Print and shaded views of the part. All mm, measured from the part's lowest x, y and z. Give positions to 0.01 mm unless a question says otherwise; leave off trailing zeros. Loops run counter-clockwise (first coordinate to the right, second up) from the corner with the lowest first, then second, coordinate; pieces in that order, holes last. Notation, with made-up numbers: M -20.5,37.5 L 24.5,37.5 A9 cw 24.5,42.5 Z; hole C -25,32 d11. An arc over 180 degrees is marked long. Answer in a Markdown table with one row per item.
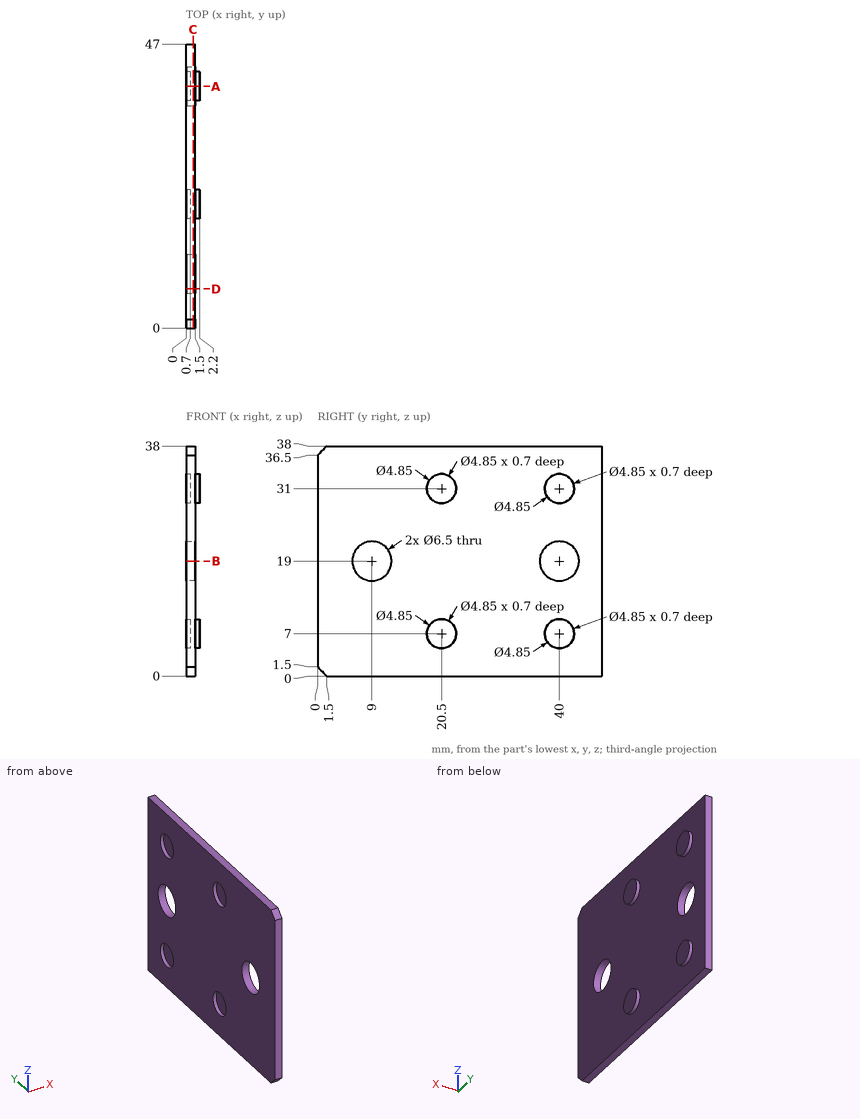
(1) Saw through at A-A, the plane y = 40. Give the cut face in (x, z) (3 decimals), and give its area (4 significant figures).
Established:
| item | result |
|---|---|
| outline | M 0,0 L 1.5,0 L 1.5,4.575 L 2.2,4.575 L 2.2,9.425 L 1.5,9.425 L 1.5,15.75 L 0,15.75 L 0,9.425 L 0.7,9.425 L 0.7,4.575 L 0,4.575 Z; M 0,22.25 L 1.5,22.25 L 1.5,28.575 L 2.2,28.575 L 2.2,33.425 L 1.5,33.425 L 1.5,38 L 0,38 L 0,33.425 L 0.7,33.425 L 0.7,28.575 L 0,28.575 Z |
| area | 47.25 mm2 |
(2) Flat gauge pins, fed straight in: P1, Ø4, axis at y = 40.5, z = 9.5, coming from the +X side; P2, Ø1.5, axis at y = 41, z = 30, coming from the -X side; P3, Ø3, axis at y = 8, z = 13, coming from the +X side. Where does each tip first touch, or does it go through?
Established:
| item | result |
|---|---|
| P1 | stops at x = 2.2 |
| P2 | stops at x = 0.7 |
| P3 | stops at x = 1.5 |
(3) Wall check: L1, parallel to Y at x = 0.45, z = 7 (3 decimals); L2, parallel to Y at x = 2.1, z = 31 (3 decimals); L3, parallel to X at y = 25, z = 30.5. Give the ranges that are in metal, low to high.
Established:
| item | result |
|---|---|
| L1 | y = 0 to 18.075, 22.925 to 37.575, 42.425 to 47 |
| L2 | y = 18.075 to 22.925, 37.575 to 42.425 |
| L3 | x = 0 to 1.5 |
(4) Saw through at D-D, the plane y = 6.5. Give the cut face in (x, z), and give its area (3 significant figures).
Established:
| item | result |
|---|---|
| outline | M 0,0 L 1.5,0 L 1.5,16.92 L 0,16.92 Z; M 0,21.08 L 1.5,21.08 L 1.5,38 L 0,38 Z |
| area | 50.8 mm2 |
(5) Saw through at C-C, the plane x = 1.15. Give the cut face in (y, z), and give its area (3 significant figures).
Established:
| item | result |
|---|---|
| outline | M 0,1.5 L 1.5,0 L 47,0 L 47,38 L 1.5,38 L 0,36.5 Z; hole C 9,19 d6.5; hole C 40,19 d6.5 |
| area | 1,720 mm2 |
(6) Saw through at B-B, the plane z = 19. Give the cut face in (x, y).
Established:
| item | result |
|---|---|
| outline | M 0,0 L 1.5,0 L 1.5,5.75 L 0,5.75 Z; M 0,12.25 L 1.5,12.25 L 1.5,36.75 L 0,36.75 Z; M 0,43.25 L 1.5,43.25 L 1.5,47 L 0,47 Z |
